from build123d import *

# Parameters (mm, degrees)
CUT_EXTRUDE1_REACH = 15.467
SKETCH2_R          = 2.325
CIRPATTERN1_COUNT  = 6


with BuildPart() as part:
    # Sketch1 → Revolve1 (revolve)
    with BuildSketch(Plane(origin=(0, 0, 0), x_dir=(0, 0, -1), z_dir=(1, 0, 0)), mode=Mode.PRIVATE) as revolve1_sk:
        Polygon((1.5, 3.1), (4.4, 3.1), (4.4, 2.1), (2.3, 2.1), (2.3, 0.5), (0, 0.5), (0, 9), (0.3, 9), (0.3, 8.7), (3.2, 8.7), (3.2, 7.75), (1.5, 7.75), align=None)
    revolve(revolve1_sk.sketch.rotate(Axis((0, 0, 59.838000458), (0, 0, -1)), 90), axis=Axis((0, 0, 59.838000458), (0, 0, -1)))

    # Sketch2 → Cut-Extrude1 (cut, up to next)
    with BuildSketch(Plane.XY, mode=Mode.PRIVATE) as cut_extrude1_sk1:
        with Locations((5.425, 0)):
            Circle(SKETCH2_R)
    cut_extrude1_tool1 = extrude(cut_extrude1_sk1.sketch, amount=-CUT_EXTRUDE1_REACH, mode=Mode.PRIVATE) & part.part
    cut_extrude1 = cut_extrude1_tool1.solids().sort_by_distance((5.425, 0, 0))[0]
    add(cut_extrude1, mode=Mode.SUBTRACT)

    # CirPattern1: Cut-Extrude1 ×6 about axis
    cirpattern1_axis = Axis((0, 0, 0), (0, 0, 1))
    for i in range(1, CIRPATTERN1_COUNT):
        add(cut_extrude1.rotate(cirpattern1_axis, i * 360 / CIRPATTERN1_COUNT), mode=Mode.SUBTRACT)


solid = part.part
Source: CAD feature listing. Evaluate the final solid. Frame: model axes, mm. A direction names the side the tool comes from. Give positions to 0.01 mm unless a question says otherwise; leave off trailing zeros. Write each loop counter-clockwise with the first axis right and the second up, starting at its lowest first coordinate (ties: lowest second). Pieces come first, ordered by that corner, then holes. Notation, with made-up numbers: M -33.75,24.5 L -15.75,24.5 A12 cw -15.75,47.5 Z; hole C 0.5,2 d4. An arc over 180 degrees is marked long. Answer as a JSON object with one key per item and string values.
Q1. Cut plane A-A, the plane z = -0.75. Count the separate pieces of the cut face and the enclosed holes in it, then the cut area to 3 significant figures.
Geometry check:
{"separate pieces": "1", "enclosed holes": "7", "area": "135 mm^2"}
Q2. Cut plane D-D, the plane x = 4.75. Return the cut outline in (y, z), then the cut area to 3 significant figures.
Geometry check:
{"outline": "M -7.64,-0.3 L -7.29,-0.3 L -7.29,-3.2 L -6.12,-3.2 L -6.12,-1.5 L -5.82,-1.5 L -5.82,0 L -7.64,0 Z; M -3.58,-1.5 L -2.22,-1.5 L -2.22,0 L -3.58,0 Z; M 2.22,-1.5 L 3.58,-1.5 L 3.58,0 L 2.22,0 Z; M 5.82,-1.5 L 6.12,-1.5 L 6.12,-3.2 L 7.29,-3.2 L 7.29,-0.3 L 7.64,-0.3 L 7.64,0 L 5.82,0 Z", "area": "12.6 mm^2"}
Q3. Cut plane B-B, the plane x = 0. Return the cut outline in (y, z), then the cut area to 3 significant figures.
Geometry check:
{"outline": "M -9,-0.3 L -8.7,-0.3 L -8.7,-3.2 L -7.75,-3.2 L -7.75,-1.5 L -3.1,-1.5 L -3.1,-4.4 L -2.1,-4.4 L -2.1,-2.3 L -0.5,-2.3 L -0.5,0 L -9,0 Z; M 0.5,-2.3 L 2.1,-2.3 L 2.1,-4.4 L 3.1,-4.4 L 3.1,-1.5 L 7.75,-1.5 L 7.75,-3.2 L 8.7,-3.2 L 8.7,-0.3 L 9,-0.3 L 9,0 L 0.5,0 Z", "area": "36.4 mm^2"}
Q4. Cut plane C-C, the plane y = 3.5. Return the cut outline in (x, z).
Geometry check:
{"outline": "M -8.29,-0.3 L -7.96,-0.3 L -7.96,-3.2 L -6.91,-3.2 L -6.91,-1.5 L -4.7,-1.5 L -4.7,0 L -8.29,0 Z; M -0.72,-1.5 L 0.72,-1.5 L 0.72,0 L -0.72,0 Z; M 4.7,-1.5 L 6.91,-1.5 L 6.91,-3.2 L 7.96,-3.2 L 7.96,-0.3 L 8.29,-0.3 L 8.29,0 L 4.7,0 Z"}
Q5. Contact query for flat-ended pins moving along their axis: P1, Ø2, axis at y = 4.5, z = -2, coming from the -X side; P2, Ø1.9, axis at x = -6, y = 4, coming from the -Z side; P3, Ø1.3, axis at x = 0.5, y = 0, coming from the -Z side. Output: stop coordinate, or through.
Geometry check:
{"P1": "stops at x = -7.96", "P2": "stops at z = -3.2", "P3": "stops at z = -2.3"}
Q6. Ray query, line 1 along Y through (x, z) = (0, -0.4); line 2 along X through (y, z) = (4.25, -1.05); line 3 along Y through (x, z) = (-4.5, -1.4). Return the intervals inside material, ascending.
Geometry check:
{"line 1": "y = -8.7 to -0.5, 0.5 to 8.7", "line 2": "x = -7.59 to -4.99, -0.43 to 0.43, 4.99 to 7.59", "line 3": "y = -7.45 to -6.18, -3.21 to -2.13, 2.13 to 3.21, 6.18 to 7.45"}
Q7. Access query for faces 1 (the face through (-1.009, -7.684, -2.338)), 2 (the face through (7.573, -0.89, -0.74)). Directions: +Z, -Z, +X, -X, +Y, -Y. A direction counts if a zero-diameter tool reaches every point of the face in a straight line with its end or side. Return the directions, or none.
Geometry check:
{"face 1": "-Z", "face 2": "+Z, -Z"}
Q8. Mould query, pull axis Y, two halves, no side actions, for faces 3 (the face through (-2, 0, 0)), 4 (the face through (-7.14, 5.48, -0.15)), 5 (the face through (-1.64, -6.76, -0.74)). Classes: +Y half, -Y half, draft (parallel to the pull), parting line (faces both ways), or undercut.
Geometry check:
{"face 3": "draft", "face 4": "parting line", "face 5": "undercut"}
